from build123d import *

# Parameters (mm, degrees)
EXTRUDE_2_DEPTH     = 70
SKETCH_3_W          = 50
SKETCH_3_H          = 25
CUT_EXTRUDE_3_DEPTH = 91


with BuildPart() as part:
    # 草图1 → 凸台-拉伸2 (new body)
    with BuildSketch(Plane.XY):
        Polygon((-42.561983471, 30.9508549), (157.438016529, 30.9508549), (157.438016529, -39.0491451), (67.438016529, -39.0491451), (67.438016529, -9.0491451), (-42.561983471, -9.0491451), align=None)
    extrude(amount=EXTRUDE_2_DEPTH)

    # 草图3 → 切除-拉伸3 (cut, through all)
    with BuildSketch(Plane.ZY.offset(-67.438016529)):
        with Locations((35, -26.5491451)):
            Rectangle(SKETCH_3_W, SKETCH_3_H)
    extrude(amount=-CUT_EXTRUDE_3_DEPTH, mode=Mode.SUBTRACT)


solid = part.part
Part model, mm, in its own coordinate system. A direction names the side the tool comes from. Give positions to 0.01 mm unless a question says otherwise; leave off trailing zeros. Loops run counter-clockwise (first coordinate to the right, second up) from the corner with the lowest first, then second, coordinate; pieces in that order, holes last. Notation, with made-up numbers: M -9.75,-18 L 45.25,-18 A13 ccw 45.25,-3 Z; hole C 64,45.5 d6. An arc over 180 degrees is marked long. Put each result on its own line as item: value. Start each with the question number.
1) Saw through at B-B (x = 118.5). List the corners of the cut face in (y, z), then the cut area to 3 significant figures.
2) Pull direction Z, two halves, no side cores. Call faces 4 (the flat face through (112, -14.049, 35)), 5 (the flat face through (-42.562, 11, 35)), 6 (the flat face through (81, 4, 70)): +Z half, -Z half, draft (parallel to the pull), parting line (faces both ways), or undercut.
3) Saw through at C-C (z = 15.5). List the corners of the cut face in (x, y).
4) Saw through at D-D (z = 7.5). List the corners of the cut face in (x, y), then the cut area to 3 significant figures.
5) Saw through at A-A (y = -23.5). List the corners of the cut face in (x, z).
6) 3-axis set-ups, long thin cutter, end or side, ignore diameter. For faces 1 (the flat face through (67.438, -13, 37)), 2 (the flat face through (112, -27, 10)), 3 (the flat face through (81, 4, 0)): which of +Z, -Z, +X, -X, +Y, -Y reach the whole face in a straight line?
7) Flat gauge pins, fed straight in: pin 1 (4 mm diameter, centred on x = 15, z = 54, fed in from -Y); pin 2 (7.5 mm diameter, centred on x = 103.5, y = -23.5, fed in from -Z). Where does each tip first touch, or does it go through?
8) Probe probe 1 along Z at (x, y) = (95, -32); probe 2 along Y at (x, z) = (114, 19); probe 3 along X at (y, z) = (-11, 40.5). List the from-to ranges inside material, lowest first.
Numbers:
1. outline: M -39.05,0 L 30.95,0 L 30.95,70 L -39.05,70 L -39.05,60 L -14.05,60 L -14.05,10 L -39.05,10 Z
1. area: 3,650 mm^2
2. face 4: undercut
2. face 5: draft
2. face 6: +Z half
3. outline: M -42.56,-9.05 L 67.44,-9.05 L 67.44,-14.05 L 157.44,-14.05 L 157.44,30.95 L -42.56,30.95 Z
4. outline: M -42.56,-9.05 L 67.44,-9.05 L 67.44,-39.05 L 157.44,-39.05 L 157.44,30.95 L -42.56,30.95 Z
4. area: 10,700 mm^2
5. outline: M 67.44,0 L 157.44,0 L 157.44,10 L 67.44,10 Z; M 67.44,60 L 157.44,60 L 157.44,70 L 67.44,70 Z
6. face 1: +Z, -Z, -X, -Y
6. face 2: +X, -X, -Y
6. face 3: -Z, +X, -X, +Y, -Y
7. pin 1: y = -9.05
7. pin 2: z = 0
8. probe 1: 0 to 10, 60 to 70
8. probe 2: -14.05 to 30.95
8. probe 3: 67.44 to 157.44
